Geometry: final body of the model. Coordinates: model frame, mm. A direction names the side the tool comes from. Give positions to 0.01 mm unless a question says otherwise; leave off trailing zeros. Loops run counter-clockwise (first coordinate to the right, second up) from the corner with the lowest first, then second, coordinate; pieces in that order, holes last.
1. First-contact query: P1, Ø1.6, axis at x = 44, z = -21.5, coming from the -Y side; P2, Ø15.5, axis at x = 17.5, y = 23, coming from the +Z side; P3, Ø1.1, axis at x = 72.5, y = 133, coming from the -Z side. Flat tips, straight axial feed; report the tip coordinate or a pass-through.
2. Section A-A, the plane x = 7. State how many separate pieces and enclosed holes the cut face has, then the cut area to 3 significant figures.
3. Section B-B, the plane y = 25. Output: boundary loops of the cut face in (x, z), then the cut area to 3 significant figures.
4. Material intervals for line 1 along Y through (x, z) = (-18.75, -11); line 2 along X through (y, z) = (124, -9.75); line 3 along Z through (x, y) = (-18.5, 458), sorted ascending.
5. Access query for faces 1 (the face through (26, 96, -22)), 2 (the face through (27.2, 167, -22.4)), 3 (the face through (-19, 227, -9)). Directions: +Z, -Z, +X, -X, +Y, -Y. A direction counts if a zero-diameter tool reaches every point of the face in a straight line with its end or side. Return the directions, or none.
6. Draft query along Z for faces 4 (the face through (73, 221, -11)), 5 (the face through (26, 440, -22)), 6 (the face through (26, 212, -22)), 7 (the face through (28, 154, -23)). Return one class per face: +Z half, -Z half, draft (parallel to the pull), parting line (faces both ways), or undercut.
from build123d import *

# Parameters (mm, degrees)
BOSS_EXTRUDE1_DEPTH = 448
SKETCH2_W           = 1
SKETCH2_H           = 20
BOSS_EXTRUDE2_DEPTH = 20
SKETCH3_W           = 1
SKETCH3_H           = 20
BOSS_EXTRUDE3_DEPTH = 20
FILLET1_R           = 2
SKETCH4_W           = 10
SKETCH4_H           = 33
CUT_EXTRUDE1_DEPTH  = 93
LPATTERN1_COUNT     = 7
LPATTERN1_PITCH     = 58
SKETCH5_R           = 2.5
CUT_EXTRUDE2_DEPTH  = 93


with BuildPart() as part:
    # Sketch1 → Boss-Extrude1 (new body)
    with BuildSketch(Plane(origin=(0, 0, 0), x_dir=(1, 0, 0), z_dir=(0, 1, 0))):
        Polygon((0, 0), (0, 1), (-18, 1), (-18, 22), (72, 22), (72, 0), (73, 0), (73, 23), (-19, 23), (-19, 0), align=None)
    extrude(amount=BOSS_EXTRUDE1_DEPTH)

    # Sketch2 → Boss-Extrude2 (add)
    with BuildSketch(Plane(origin=(0, 448, 0), x_dir=(1, 0, 0), z_dir=(0, 1, 0))):
        with Locations((-18.5, 11)):
            Rectangle(SKETCH2_W, SKETCH2_H)
        with Locations((72.5, 11)):
            Rectangle(SKETCH2_W, SKETCH2_H)
    extrude(amount=BOSS_EXTRUDE2_DEPTH)

    # Sketch3 → Boss-Extrude3 (add)
    with BuildSketch(Plane(origin=(0, 0, 0), x_dir=(-1, 0, 0), z_dir=(0, -1, 0))):
        with Locations((18.5, 11)):
            Rectangle(SKETCH3_W, SKETCH3_H)
        with Locations((-72.5, 11)):
            Rectangle(SKETCH3_W, SKETCH3_H)
    extrude(amount=BOSS_EXTRUDE3_DEPTH)

    # Fillet1
    fillet1_edges = [part.edges().sort_by_distance(p)[0] for p in [
        (-18.5, 468, -21),
        (-18.5, 468, -1),
        (72.5, 468, -1),
        (72.5, 468, -21),
        (-18.5, -20, -1),
        (-18.5, -20, -21),
        (72.5, -20, -21),
        (72.5, -20, -1),
    ]]
    fillet(fillet1_edges, radius=FILLET1_R)

    # Sketch4 → Cut-Extrude1 (cut, through all)
    with BuildSketch(Plane(origin=(73, 0, 0), x_dir=(0, 0, -1), z_dir=(1, 0, 0))):
        with Locations((18, 415.5)):
            Rectangle(SKETCH4_W, SKETCH4_H)
    cut_extrude1 = extrude(amount=-CUT_EXTRUDE1_DEPTH, mode=Mode.SUBTRACT)

    # LPattern1: Cut-Extrude1 ×7
    with Locations(*[(0, -i * LPATTERN1_PITCH, 0) for i in range(1, LPATTERN1_COUNT)]):
        add(cut_extrude1, mode=Mode.SUBTRACT)

    # Sketch5 → Cut-Extrude2 (cut, through all)
    with BuildSketch(Plane(origin=(73, 0, 0), x_dir=(0, 0, -1), z_dir=(1, 0, 0))):
        with Locations((11, 458)):
            Circle(SKETCH5_R)
        with Locations((11, -10)):
            Circle(SKETCH5_R)
    extrude(amount=-CUT_EXTRUDE2_DEPTH, mode=Mode.SUBTRACT)


solid = part.part
Answers below:
1. P1: stops at y = 0
1. P2: stops at z = -22
1. P3: stops at z = -13
2. separate pieces: 8
2. enclosed holes: 0
2. area: 217 mm2
3. outline: (-19, -23) - (73, -23) - (73, 0) - (72, 0) - (72, -22) - (-18, -22) - (-18, -1) - (0, -1) - (0, 0) - (-19, 0) - close
3. area: 154 mm2
4. line 1: y = -20 to -12.5, -7.5 to 455.5, 460.5 to 468
4. line 2: x = -19 to -18, 72 to 73
4. line 3: z = -21 to -13.5, -8.5 to -1
5. face 1: +Y, -Y
5. face 2: -Z, +X, -X
5. face 3: +Z, -Z, -X, +Y, -Y
6. face 4: draft
6. face 5: undercut
6. face 6: undercut
6. face 7: -Z half
